The drawing under review shows one solid part. Ordinate dimensions are in mm from its lowest x, y, z. A direction names the side the tool comes from. Coordinates: 2 decimals unless noted, no trailing zeros. Order: outer loops, then holes, each group sorted by start corner. A loop starts at its lowest first (then second) coordinate and runs counter-clockwise, first axis right, second up.
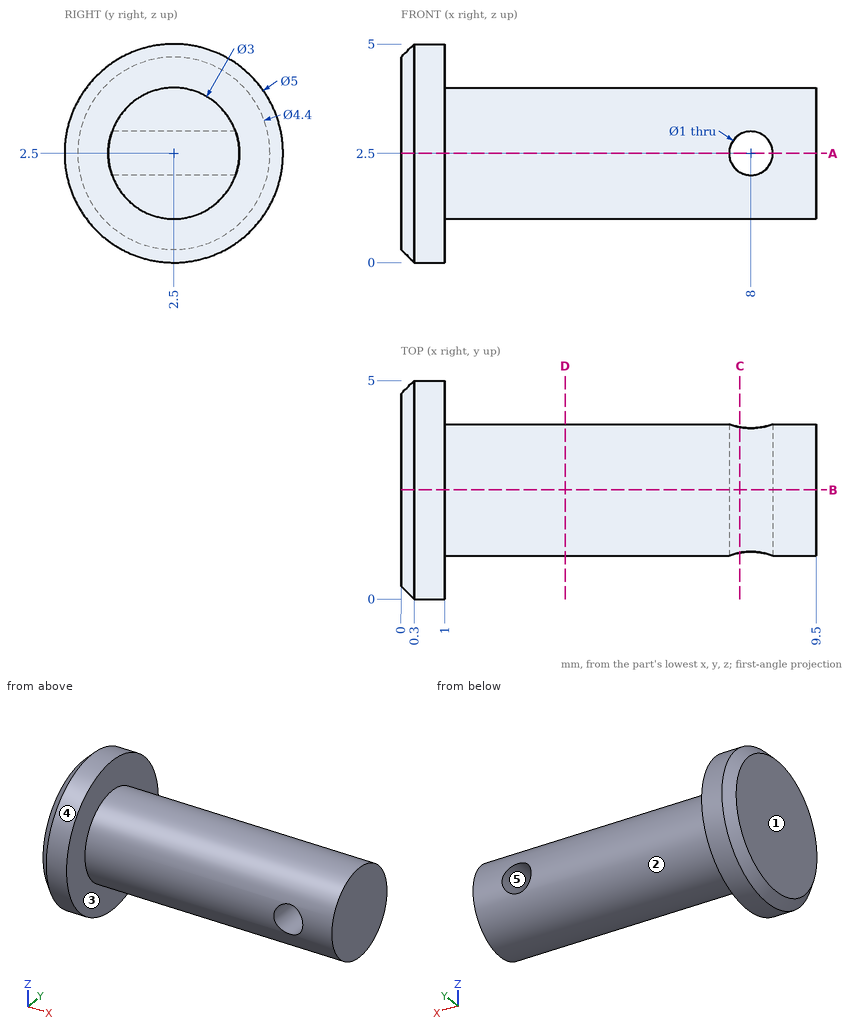
1. Take a section at C-C, the plane x = 7.75. Give the boundary of the cut face in (y, z).
Answer below:
outline: (1.06, 2.07) arc R1.5 ccw to (3.94, 2.07) - close; (1.06, 2.93) - (3.94, 2.93) arc R1.5 ccw to start
2. The part is to be moulded in two halves that separate along X. For the marked faces 3, 4 and 5, say which applies: +X half, -X half, draft (parallel to the pull), parting line (faces both ways), or undercut.
Answer below:
face 3: +X half
face 4: draft
face 5: undercut
3. Clearance check with flat-ended pins moving along their axes: pin 1 Ø3 at (x, z) = (7.5, 2.5) entering from -Y; pin 2 Ø2 at (x, y) = (6.5, 0.5) entering from -Z. State where each tip first meets the part, or that it passes through.
Answer below:
pin 1: stops at y = 1
pin 2: stops at z = 1.38
4. Take a section at D-D, the plane x = 3.75. Give the boundary of the cut face in (y, z).
Answer below:
outline: circle Ø3 at (2.5, 2.5)
5. Machinability: for the marked faces 1 and 2, which of the approach directions +Z, -Z, +X, -X, +Y, -Y give a long, thin tool a straight path to every point of the face, cutting with its end or side? Answer none if there is none.
Answer below:
face 1: +Z, -Z, -X, +Y, -Y
face 2: +X
6. Take a section at A-A, the plane z = 2.5. Give the boundary of the cut face in (x, y), plus the area to 3 significant figures.
Answer below:
outline: (0, 0.3) - (0.3, 0) - (1, 0) - (1, 1) - (7.5, 1) - (7.5, 4) - (1, 4) - (1, 5) - (0.3, 5) - (0, 4.7) - close; (8.5, 1) - (9.5, 1) - (9.5, 4) - (8.5, 4) - close
area: 27.4 mm2
7. Take a section at B-B, the plane y = 2.5. Give the boundary of the cut face in (x, z).
Answer below:
outline: (0, 0.3) - (0.3, 0) - (1, 0) - (1, 1) - (9.5, 1) - (9.5, 4) - (1, 4) - (1, 5) - (0.3, 5) - (0, 4.7) - close; hole circle Ø1 at (8, 2.5)
8. To check wall thickness, follow L1, parallel to X at y = 2.4, z = 2.5; L2, parallel to Z at x = 8, y = 2.5; L3, parallel to Z at x = 8, y = 3.35. State the ranges of each line that lie inside material, in increasing order.
Answer below:
L1: x = 0 to 7.5, 8.5 to 9.5
L2: z = 1 to 2, 3 to 4
L3: z = 1.26 to 2, 3 to 3.74
